Check sheet for the modelled part. Datum: model origin and axes. Units: mm. A direction names the side the tool comes from. Give positions to 0.01 mm unless a question says otherwise; leave off trailing zeros. Loops run counter-clockwise (first coordinate to the right, second up) from the corner with the lowest first, then second, coordinate; pieces in that order, holes last. Notation, with made-up numbers: (-23.75, 56.5) -> (27.25, 56.5) arc R13 cw to (27.25, 61.5) -> close; hole circle Ø7 at (48.5, 88.5). An arc over 180 degrees is marked (long way). Write each question's results on one line, items separated by ' | '. Start each with the question number.
Item 1: Cross-section at B-B on y = -11. Enter the section's corners in (x, z).
Item 2: Access from +Z, -Z, +X, -X, +Y, -Y to the whole of each face (thin tool, end or side, straight path). Record for faces 5 (the face through (-15.378, -12, 10)), 6 (the face through (7, -14, 7.253)), 7 (the face through (-1.65, -26.27, 10.21)).
Item 3: Cross-section at D-D on y = -26. Enter the section's corners in (x, z).
Item 4: Scan lines: line 1 along X through (y, z) = (-9, 9.5); line 2 along X through (y, z) = (-9, 14.75); line 3 along X through (y, z) = (-13, 17.25). Record each from-to range of solid material in increasing order.
Item 5: Gauge pin test, flat end, axial feed: pin 1 Ø6 at (x, z) = (-26.5, 13) entering from -Y. Record the tip position at first contact, or that the pin passes through.
Item 6: Mould release check, pull along X, two halves, no side actions. Record for faces 1 (the face through (-5.378, -12, 10)), 2 (the face through (-10.83, -30, 20.34)), 3 (the face through (-11.65, -26.27, 10.21)), 4 (the face through (29.622, -15, 15)): pulls with the +X half, pulls with the -X half, needs draft (parallel to the pull), parting line crosses it, or undercut.
Item 7: Cross-section at A-A on y = -15. State how many separate pieces and enclosed holes the cut face has, then the cut area to 3 significant figures.
from build123d import *

# Parameters (mm, degrees)
F1_DEPTH     = 30
F3_D         = 6
F4_T1_DEPTH  = 18.8584149398
F4_T4_ANGLE  = 180
F4_T6_ANGLE  = 180
F4_T8_ANGLE  = 180
F4_T10_ANGLE = 180
F4_T12_ANGLE = 180


# Not quite as in the source:
# - a fillet or chamfer that OpenCascade refuses, or shapes differently, is made with other operations: its cross-section is extruded or revolved along the edge and cut away or added


with BuildPart() as f1:
    # F0 (on Front) → F1 (new body)
    with BuildSketch(Plane.XZ):
        with BuildLine():
            Line((29.6215080619, 22.2534802178), (-45.3784919381, 22.2534802178))
            Line((-45.3784919381, 22.2534802178), (-45.3784919381, 7.2534802178))
            Line((-45.3784919381, 7.2534802178), (-30.3784919381, 7.2534802178))
            Line((-30.3784919381, 7.2534802178), (-30.3784919381, 13.2534802178))
            ThreePointArc((-30.3784919381, 13.2534802178), (-27.8784919381, 15.7534802178), (-25.3784919381, 13.2534802178))
            Line((-25.3784919381, 13.2534802178), (-25.3784919381, 7.2534802178))
            Line((-25.3784919381, 7.2534802178), (-20.3784919381, 7.2534802178))
            Line((-20.3784919381, 7.2534802178), (-20.3784919381, 13.2534802178))
            ThreePointArc((-20.3784919381, 13.2534802178), (-17.8784919381, 15.7534802178), (-15.3784919381, 13.2534802178))
            Line((-15.3784919381, 13.2534802178), (-15.3784919381, 7.2534802178))
            Line((-15.3784919381, 7.2534802178), (-10.3784919381, 7.2534802178))
            Line((-10.3784919381, 7.2534802178), (-10.3784919381, 13.2534802178))
            ThreePointArc((-10.3784919381, 13.2534802178), (-7.8784919381, 15.7534802178), (-5.3784919381, 13.2534802178))
            Line((-5.3784919381, 13.2534802178), (-5.3784919381, 7.2534802178))
            Line((-5.3784919381, 7.2534802178), (-0.3784919381, 7.2534802178))
            Line((-0.3784919381, 7.2534802178), (-0.3784919381, 13.2534802178))
            ThreePointArc((-0.3784919381, 13.2534802178), (2.1215080619, 15.7534802178), (4.6215080619, 13.2534802178))
            Line((4.6215080619, 13.2534802178), (4.6215080619, 7.2534802178))
            Line((4.6215080619, 7.2534802178), (9.6215080619, 7.2534802178))
            Line((9.6215080619, 7.2534802178), (9.6215080619, 13.2534802178))
            ThreePointArc((9.6215080619, 13.2534802178), (12.1215080619, 15.7534802178), (14.6215080619, 13.2534802178))
            Line((14.6215080619, 13.2534802178), (14.6215080619, 7.2534802178))
            Line((14.6215080619, 7.2534802178), (29.6215080619, 7.2534802178))
            Line((29.6215080619, 7.2534802178), (29.6215080619, 22.2534802178))
        make_face()
    extrude(amount=F1_DEPTH)

    # F3 (through all)
    with Locations(Plane.XY.offset(22.2534802178)):
        with Locations((-37.3784919381, -15), (21.6215080619, -15)):
            Hole(F3_D / 2)

    # F4: chamfer of 5 on 5 edges, made by hand

    # F4_s2 → F4_t1 (cut)
    with BuildSketch(Plane.XY.offset(-5.604934722)):
        Polygon((-35.3784919381, -30), (-30.3784919381, -25), (-30.3784919381, -30), align=None)
        Polygon((-25.3784919381, -30), (-20.3784919381, -25), (-20.3784919381, -30), align=None)
        Polygon((-15.3784919381, -30), (-10.3784919381, -25), (-10.3784919381, -30), align=None)
        Polygon((-5.3784919381, -30), (-0.3784919381, -25), (-0.3784919381, -30), align=None)
        Polygon((4.6215080619, -30), (9.6215080619, -25), (9.6215080619, -30), align=None)
        Polygon((19.6215080619, -30), (14.6215080619, -25), (14.6215080619, -30), align=None)
        Polygon((9.6215080619, -30), (4.6215080619, -25), (4.6215080619, -30), align=None)
        Polygon((-0.3784919381, -30), (-5.3784919381, -25), (-5.3784919381, -30), align=None)
        Polygon((-10.3784919381, -30), (-15.3784919381, -25), (-15.3784919381, -30), align=None)
        Polygon((-20.3784919381, -30), (-25.3784919381, -25), (-25.3784919381, -30), align=None)
    extrude(amount=F4_T1_DEPTH, mode=Mode.SUBTRACT)

    # F4_s3 → F4_t4 (revolve, cut)
    with BuildSketch(Plane.XY.offset(13.2534802178)):
        Polygon((4.6215080619, -30), (9.6215080619, -25), (9.6215080619, -30), align=None)
    revolve(axis=Axis((12.1215080619, -30, 13.2534802178), (0, 1, 0)), revolution_arc=F4_T4_ANGLE, mode=Mode.SUBTRACT)

    # F4_s5 → F4_t6 (revolve, cut)
    with BuildSketch(Plane.XY.offset(13.2534802178)):
        Polygon((-5.3784919381, -30), (-0.3784919381, -25), (-0.3784919381, -30), align=None)
    revolve(axis=Axis((2.1215080619, -30, 13.2534802178), (0, 1, 0)), revolution_arc=F4_T6_ANGLE, mode=Mode.SUBTRACT)

    # F4_s7 → F4_t8 (revolve, cut)
    with BuildSketch(Plane.XY.offset(13.2534802178)):
        Polygon((-15.3784919381, -30), (-10.3784919381, -25), (-10.3784919381, -30), align=None)
    revolve(axis=Axis((-7.8784919381, -30, 13.2534802178), (0, 1, 0)), revolution_arc=F4_T8_ANGLE, mode=Mode.SUBTRACT)

    # F4_s9 → F4_t10 (revolve, cut)
    with BuildSketch(Plane.XY.offset(13.2534802178)):
        Polygon((-25.3784919381, -30), (-20.3784919381, -25), (-20.3784919381, -30), align=None)
    revolve(axis=Axis((-17.8784919381, -30, 13.2534802178), (0, 1, 0)), revolution_arc=F4_T10_ANGLE, mode=Mode.SUBTRACT)

    # F4_s11 → F4_t12 (revolve, cut)
    with BuildSketch(Plane.XY.offset(13.2534802178)):
        Polygon((-35.3784919381, -30), (-30.3784919381, -25), (-30.3784919381, -30), align=None)
    revolve(axis=Axis((-27.8784919381, -30, 13.2534802178), (0, 1, 0)), revolution_arc=F4_T12_ANGLE, mode=Mode.SUBTRACT)


solid = f1.part
Answer sheet:
1) outline: (-45.38, 7.25) -> (-30.38, 7.25) -> (-30.38, 13.25) arc R2.5 cw to (-25.38, 13.25) -> (-25.38, 7.25) -> (-20.38, 7.25) -> (-20.38, 13.25) arc R2.5 cw to (-15.38, 13.25) -> (-15.38, 7.25) -> (-10.38, 7.25) -> (-10.38, 13.25) arc R2.5 cw to (-5.38, 13.25) -> (-5.38, 7.25) -> (-0.38, 7.25) -> (-0.38, 13.25) arc R2.5 cw to (4.62, 13.25) -> (4.62, 7.25) -> (9.62, 7.25) -> (9.62, 13.25) arc R2.5 cw to (14.62, 13.25) -> (14.62, 7.25) -> (29.62, 7.25) -> (29.62, 22.25) -> (-45.38, 22.25) -> close
2) face 5: -Z, +Y, -Y | face 6: -Z, +X, -X, +Y, -Y | face 7: -Z, -Y
3) outline: (-45.38, 7.25) -> (-31.38, 7.25) -> (-31.38, 13.25) arc R3.5 cw to (-24.38, 13.25) -> (-24.38, 7.25) -> (-21.38, 7.25) -> (-21.38, 13.25) arc R3.5 cw to (-14.38, 13.25) -> (-14.38, 7.25) -> (-11.38, 7.25) -> (-11.38, 13.25) arc R3.5 cw to (-4.38, 13.25) -> (-4.38, 7.25) -> (-1.38, 7.25) -> (-1.38, 13.25) arc R3.5 cw to (5.62, 13.25) -> (5.62, 7.25) -> (8.62, 7.25) -> (8.62, 13.25) arc R3.5 cw to (15.62, 13.25) -> (15.62, 7.25) -> (29.62, 7.25) -> (29.62, 22.25) -> (-45.38, 22.25) -> close
4) line 1: x = -45.38 to -30.38, -25.38 to -20.38, -15.38 to -10.38, -5.38 to -0.38, 4.62 to 9.62, 14.62 to 29.62 | line 2: x = -45.38 to -29.88, -25.88 to -19.88, -15.88 to -9.88, -5.88 to 0.12, 4.12 to 10.12, 14.12 to 29.62 | line 3: x = -45.38 to -39.61, -35.14 to 19.39, 23.86 to 29.62
5) pin 1: stops at y = -26.88
6) face 1: undercut | face 2: needs draft | face 3: undercut | face 4: pulls with the +X half
7) separate pieces: 3 | enclosed holes: 0 | area: 746 mm²
